For this review, use the dimensioned drawing (mm, ordinates from the lowest corner) and the shaded views. Coordinates: 2 decimals unless noted, no trailing zeros. Write each loop counter-clockwise with the first axis right and the second up, starting at its lowest first coordinate (ties: lowest second). Pieces come first, ordered by that corner, then holes. Notation, with made-up numbers: (85.5, -26.75) - (128.5, -26.75) arc R27 cw to (128.5, 4.25) - close; hole circle Ø5 at (-14, -6). An arc over 180 degrees is marked (long way). One line per item, written item: value.
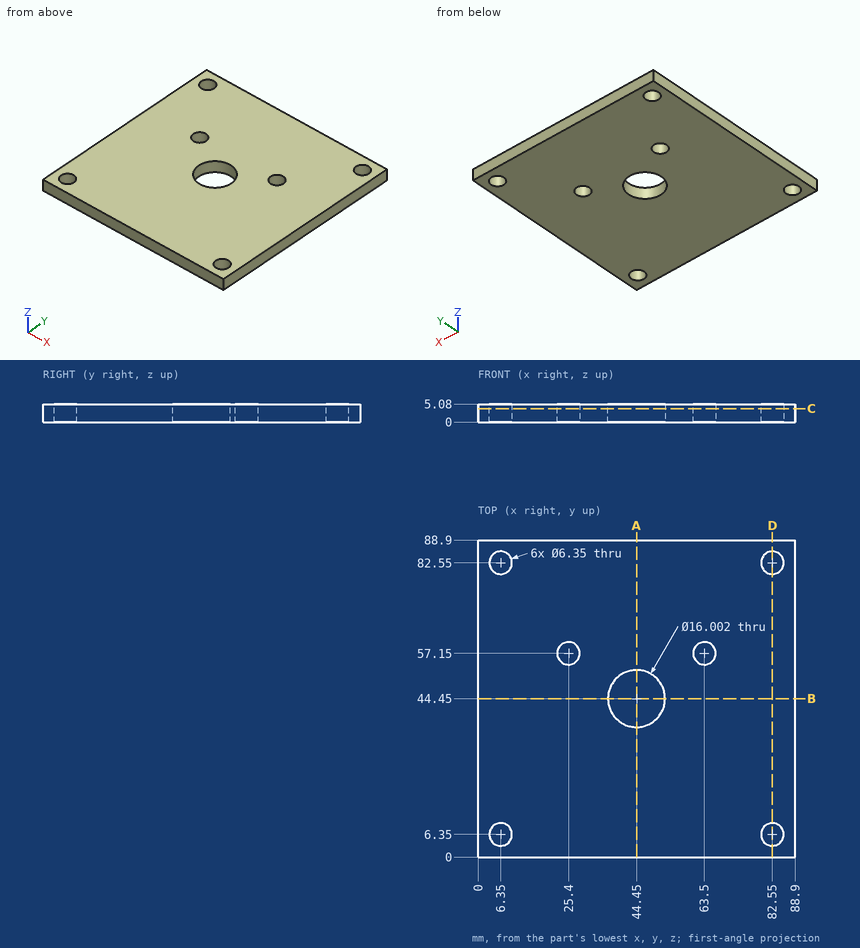
1. Consider section C-C, the plane z = 3.8. Write out the cut boundary in (x, y) (3 decimals), then the cut area to 3 significant figures.
Answer block:
outline: (0, 0) - (88.9, 0) - (88.9, 88.9) - (0, 88.9) - close; hole circle Ø6.35 at (6.35, 6.35); hole circle Ø6.35 at (6.35, 82.55); hole circle Ø6.35 at (25.4, 57.15); hole circle Ø16.002 at (44.45, 44.45); hole circle Ø6.35 at (63.5, 57.15); hole circle Ø6.35 at (82.55, 6.35); hole circle Ø6.35 at (82.55, 82.55)
area: 7,510 mm^2
2. Insertion check: pin 1 Ø8.5 at (x, y) = (63.5, 57.15) entering from -Z; pin 2 Ø5.5 at (x, y) = (82.55, 6.35) entering from -Z. Each pin has a flat end and moves straight along its axis. Give the tip position at first contact, or say it passes through.
Answer block:
pin 1: stops at z = 0
pin 2: passes through
3. Wall thickness on line 1 along Y through (x, z) = (6.35, 3.8) (3 decimals); line 2 along X through (y, z) = (6, 2.3); line 3 along Y through (x, z) = (44.45, 1.85): over which ranges is each line inside the solid? List them lowest first.
Answer block:
line 1: y = 0 to 3.175, 9.525 to 79.375, 85.725 to 88.9
line 2: x = 0 to 3.19, 9.51 to 79.39, 85.71 to 88.9
line 3: y = 0 to 36.45, 52.45 to 88.9
4. Consider section A-A, the plane x = 44.45. Write out the cut boundary in (y, z), then the cut area to 3 significant figures.
Answer block:
outline: (0, 0) - (36.45, 0) - (36.45, 5.08) - (0, 5.08) - close; (52.45, 0) - (88.9, 0) - (88.9, 5.08) - (52.45, 5.08) - close
area: 370 mm^2
5. Consider section D-D, the plane x = 82.55. Write out the cut boundary in (y, z) (3 decimals).
Answer block:
outline: (0, 0) - (3.175, 0) - (3.175, 5.08) - (0, 5.08) - close; (9.525, 0) - (79.375, 0) - (79.375, 5.08) - (9.525, 5.08) - close; (85.725, 0) - (88.9, 0) - (88.9, 5.08) - (85.725, 5.08) - close
